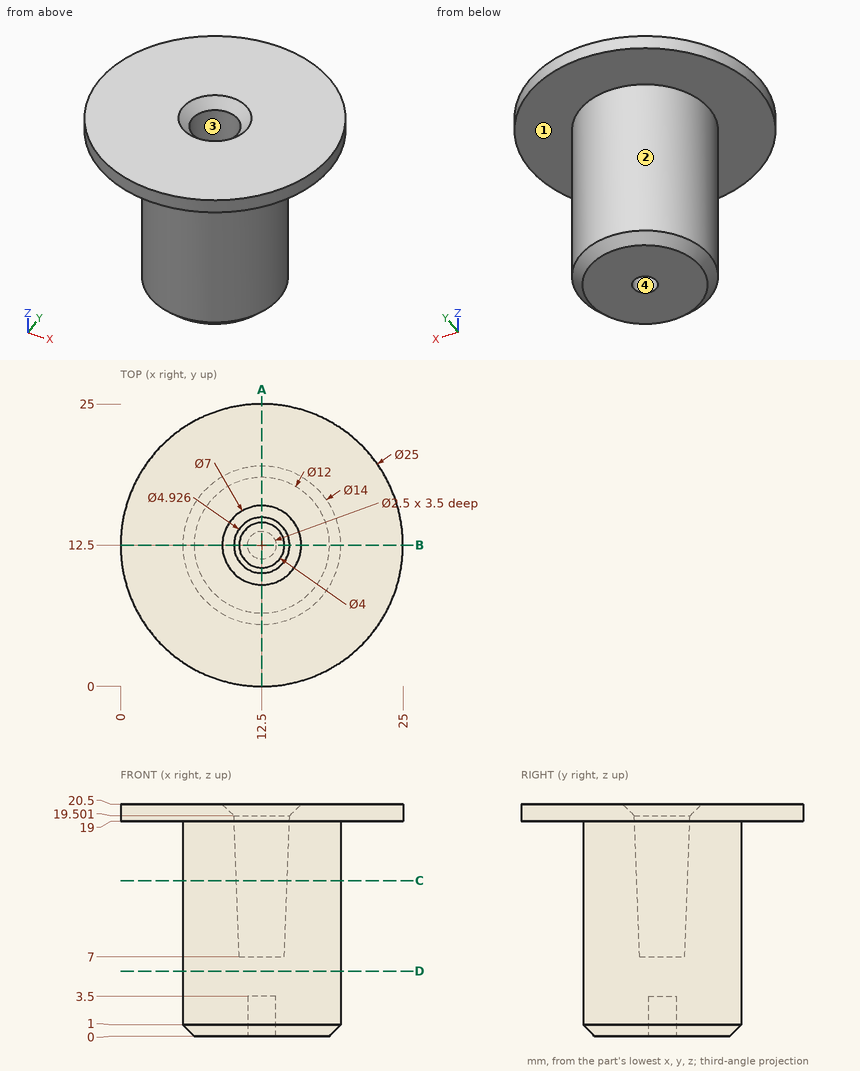
Input: dimensioned drawing with shaded views. Units: mm. Origin: part minimum x, y, z. Coordinates: 2 decimals unless noted, no trailing zeros. Write each loop counter-clockwise with the first axis right and the second up, starting at its lowest first coordinate (ties: lowest second). Pieces come first, ordered by that corner, then holes. Notation, with made-up numbers: M 51,84 L 56,84 A29 ccw 56,118 Z; hole C -19,37.25 d9. An arc over 180 degrees is marked long. Answer as CSV lines item,"result". Start each with the question number.
Q1. Cut plane A-A on x = 12.5. Return the cut outline in (y, z), then the cut area to 3 significant figures.
Q2. Mould query, pull axis X, two halves, no side actions, for the marked faces 1, 2, 3 and 4. Classes: released by +X, released by -X, zero draft, split by the parting line, or undercut.
Q3. Line query: line 1 (X direction, y = 12.5, z = 2.55); line 2 (Z direction, x = 13.5, y = 21.5). Output: solid intervals per line, ascending. Write a range as from..to.
Q4. Cut plane D-D on z = 5.75. Return the cut outline in (x, y), then the cut area to 3 significant figures.
Q5. Pin query (flat end, axial travel): P1, Ø1.5, axis at x = 17, z = 8.5, coming from the +Y side; P2, Ø2, axis at x = 12.5, z = 15.5, coming from the +Y side; P3, Ø1, axis at x = 21.5, z = 15.5, coming from the -Y side; P4, Ø10, axis at x = 4, z = 3, coming from the -Y side. Return the tip coordinate at first contact, or that it passes through.
Q6. Cut plane C-C on z = 13.75. Return the cut outline in (x, y), then the cut area to 3 significant figures.
Findings below:
1,outline,"M 0,19 L 5.5,19 L 5.5,1 L 6.5,0 L 11.25,0 L 11.25,3.5 L 13.75,3.5 L 13.75,0 L 18.5,0 L 19.5,1 L 19.5,19 L 25,19 L 25,20.5 L 16,20.5 L 14.96,19.5 L 14.5,7 L 10.5,7 L 10.04,19.5 L 9,20.5 L 0,20.5 Z"
1,area,"232 mm2"
2,face 1,"zero draft"
2,face 2,"split by the parting line"
2,face 3,"undercut"
2,face 4,"undercut"
3,line 1,"x = 5.5..11.25, 13.75..19.5"
3,line 2,"z = 19..20.5"
4,outline,"C 12.5,12.5 d14"
4,area,"154 mm2"
5,P1,"stops at y = 18.41"
5,P2,"stops at y = 19.5"
5,P3,"passes through"
5,P4,"stops at y = 6.44"
6,outline,"C 12.5,12.5 d14; hole C 12.5,12.5 d4.5"
6,area,"138 mm2"
